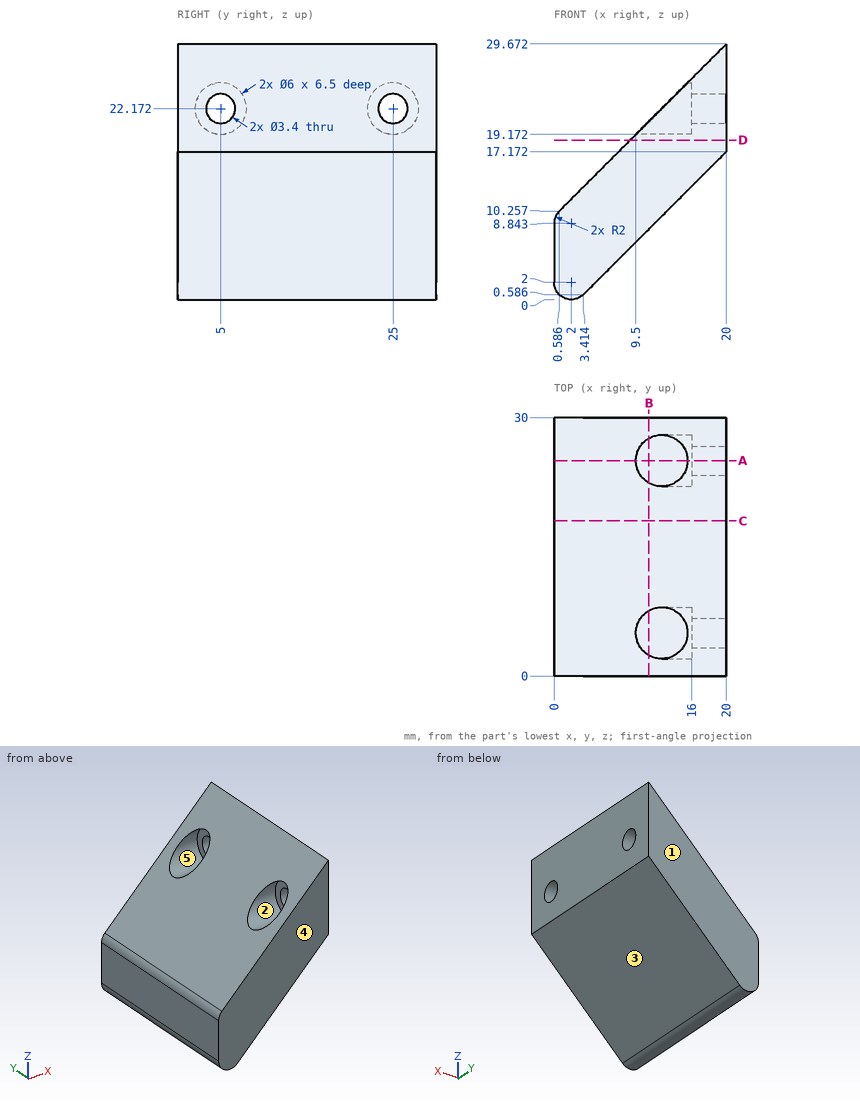
Geometry: see drawing. Coordinates: mm, zero at the bounding-box minimum. A direction names the side the tool comes from. Round coordinates to 2 decimals unless told otherwise and drop trailing zeros. Order: outer loops, then holes, each group sorted by start corner. A loop starts at its lowest first (then second) coordinate and runs counter-clockwise, first axis right, second up. Notation, with made-up numbers: (79.25, 11.5) -> (121.25, 11.5) arc R36 ccw to (121.25, 48.5) -> close; hole circle Ø11 at (-26.75, 43.25). An arc over 180 degrees is marked (long way). Write each question's results on one line, items separated by ' | '.
Q1. Section query B-B (x = 11). Output: boundary loops of the cut face in (y, z), and give its area (3 significant figures).
Response values:
outline: (0, 8.17) -> (30, 8.17) -> (30, 20.67) -> (27.6, 20.67) arc R3 cw to (22.4, 20.67) -> (7.6, 20.67) arc R3 cw to (2.4, 20.67) -> (0, 20.67) -> close | area: 364 mm²
Q2. Access query for the marked faces 4 and 5. Directions: +Z, -Z, +X, -X, +Y, -Y. A direction counts if a zero-diameter tool reaches every point of the face in a straight line with its end or side. Return the directions, or none.
Response values:
face 4: +Z, -Z, +X, -X, -Y | face 5: -X
Q3. Section query D-D (z = 18.5). Output: boundary loops of the cut face in (x, y).
Response values:
outline: (8.83, 0) -> (20, 0) -> (20, 30) -> (8.83, 30) -> close
Q4. Section query C-C (y = 18). Output: boundary loops of the cut face in (x, z) (1 decimal).
Response values:
outline: (0, 2) arc R2 ccw to (3.4, 0.6) -> (20, 17.2) -> (20, 29.7) -> (0.6, 10.3) arc R2 ccw to (0, 8.8) -> close
Q5. Pin query (flat end, axial travel): pin 1 Ø2 at (y, z) = (25, 22.17) entering from -X; pin 2 Ø4 at (y, z) = (5, 22.17) entering from -X; pin 3 Ø5 at (y, z) = (4.5, 21.5) entering from -X; pin 4 Ø1.5 at (x, y) = (14, 25) entering from -Z. Return the tip coordinate at first contact, or that it passes through.
Response values:
pin 1: through | pin 2: x = 16 | pin 3: x = 9.33 | pin 4: z = 10.42
Q6. Ray query, line 1 along Y through (x, z) = (14.25, 22) (1 decimal); line 2 along Y through (x, z) = (19, 23.25) (1 decimal); line 3 along Z through (x, y) = (11.25, 8.25). Return the intervals inside material, ascending.
Response values:
line 1: 0 to 2, 8 to 22, 28 to 30 | line 2: 0 to 3.7, 6.3 to 23.7, 26.3 to 30 | line 3: 8.42 to 20.92
Q7. Pull-direction query (Y, two-part tool) for the marked faces 1, 2 and 3; classes: released by +Y, released by -Y, zero draft, split by the parting line, or undercut.
Response values:
face 1: released by +Y | face 2: undercut | face 3: zero draft
Q8. Section query A-A (y = 25). Output: boundary loops of the cut face in (x, z) (1 decimal).
Response values:
outline: (0, 2) arc R2 ccw to (3.4, 0.6) -> (20, 17.2) -> (20, 20.5) -> (16, 20.5) -> (16, 19.2) -> (9.5, 19.2) -> (0.6, 10.3) arc R2 ccw to (0, 8.8) -> close; (15.5, 25.2) -> (16, 25.2) -> (16, 23.9) -> (20, 23.9) -> (20, 29.7) -> close
